Autodesk Fusion 360 part; units mm, degrees
sketch "Eskiz1" plane through (0, 0, 0) normal (0, 1, 0) x (1, 0, 0)
  circle A0 centre (0, 0) radius 20
  circle A1 centre (0, 0) radius 50
  line L0 (-5, 44.3809) -> (5, 44.3809)
  line L1 (5, 44.3809) -> (5, 24.3809)
  line L2 (5, 24.3809) -> (-5, 24.3809)
  line L3 (-5, 24.3809) -> (-5, 44.3809)
  circle A2 centre (-5, 24.3809) radius 1.5
  circle A3 centre (5, 24.3809) radius 1.5
  circle A4 centre (-5, 44.3809) radius 1.5
  circle A5 centre (5, 44.3809) radius 1.5
  circle A6 centre (-34.9176, 27.8465) radius 1.5
  line L4 (-34.9176, 27.8465) -> (-27.8465, 34.9176)
  line L5 (-20.7754, 13.7044) -> (-34.9176, 27.8465)
  line L6 (-13.7044, 20.7754) -> (-20.7754, 13.7044)
  line L7 (-27.8465, 34.9176) -> (-13.7044, 20.7754)
  circle A7 centre (-27.8465, 34.9176) radius 1.5
  circle A8 centre (-20.7754, 13.7044) radius 1.5
  circle A9 centre (-13.7044, 20.7754) radius 1.5
  circle A10 centre (-44.3809, -5) radius 1.5
  line L8 (-44.3809, -5) -> (-44.3809, 5)
  line L9 (-24.3809, -5) -> (-44.3809, -5)
  line L10 (-24.3809, 5) -> (-24.3809, -5)
  line L11 (-44.3809, 5) -> (-24.3809, 5)
  circle A11 centre (-44.3809, 5) radius 1.5
  circle A12 centre (-24.3809, -5) radius 1.5
  circle A13 centre (-24.3809, 5) radius 1.5
  circle A14 centre (-27.8465, -34.9176) radius 1.5
  line L12 (-27.8465, -34.9176) -> (-34.9176, -27.8465)
  line L13 (-13.7044, -20.7754) -> (-27.8465, -34.9176)
  line L14 (-20.7754, -13.7044) -> (-13.7044, -20.7754)
  line L15 (-34.9176, -27.8465) -> (-20.7754, -13.7044)
  circle A15 centre (-34.9176, -27.8465) radius 1.5
  circle A16 centre (-13.7044, -20.7754) radius 1.5
  circle A17 centre (-20.7754, -13.7044) radius 1.5
  circle A18 centre (5, -44.3809) radius 1.5
  line L16 (5, -44.3809) -> (-5, -44.3809)
  line L17 (5, -24.3809) -> (5, -44.3809)
  line L18 (-5, -24.3809) -> (5, -24.3809)
  line L19 (-5, -44.3809) -> (-5, -24.3809)
  circle A19 centre (-5, -44.3809) radius 1.5
  circle A20 centre (5, -24.3809) radius 1.5
  circle A21 centre (-5, -24.3809) radius 1.5
  circle A22 centre (34.9176, -27.8465) radius 1.5
  line L20 (34.9176, -27.8465) -> (27.8465, -34.9176)
  line L21 (20.7754, -13.7044) -> (34.9176, -27.8465)
  line L22 (13.7044, -20.7754) -> (20.7754, -13.7044)
  line L23 (27.8465, -34.9176) -> (13.7044, -20.7754)
  circle A23 centre (27.8465, -34.9176) radius 1.5
  circle A24 centre (20.7754, -13.7044) radius 1.5
  circle A25 centre (13.7044, -20.7754) radius 1.5
  circle A26 centre (44.3809, 5) radius 1.5
  line L24 (44.3809, 5) -> (44.3809, -5)
  line L25 (24.3809, 5) -> (44.3809, 5)
  line L26 (24.3809, -5) -> (24.3809, 5)
  line L27 (44.3809, -5) -> (24.3809, -5)
  circle A27 centre (44.3809, -5) radius 1.5
  circle A28 centre (24.3809, 5) radius 1.5
  circle A29 centre (24.3809, -5) radius 1.5
  circle A30 centre (27.8465, 34.9176) radius 1.5
  line L28 (27.8465, 34.9176) -> (34.9176, 27.8465)
  line L29 (13.7044, 20.7754) -> (27.8465, 34.9176)
  line L30 (20.7754, 13.7044) -> (13.7044, 20.7754)
  line L31 (34.9176, 27.8465) -> (20.7754, 13.7044)
  circle A31 centre (34.9176, 27.8465) radius 1.5
  circle A32 centre (13.7044, 20.7754) radius 1.5
  circle A33 centre (20.7754, 13.7044) radius 1.5
  circle A34 centre (0, 0) radius 3.9
  point P0 (-5, 0)
  point P1 (5, 0)
  dimension "d1" = 40
  dimension "d2" = 100
  dimension "d3" = 5
  dimension "d4" = 5
  dimension "d5" = 10
  dimension "d6" = 20
  dimension "d9" = 44.3809
  dimension "d10" = 3
  dimension "d11" = 3
  dimension "d12" = 3
  dimension "d13" = 3
  dimension "d15" = 360
  dimension "d16" = 7.8
extrude "Ekstrüde Et1" add sketch "Eskiz1" along normal blind 10 contours A0 | A1
extrude "Ekstrüde Et2" add sketch "Eskiz1" along normal blind 6.5 contours A0
sketch "Eskiz2" plane through (0, 10, 0) normal (0, 1, 0) x (-1, 0, 0)
  arc A0 (-14.765, -21.8361) -> (-14.765, -19.7148) centre (-13.7044, -20.7754) ccw
  line L0 (-14.765, -21.8361) -> (-26.7858, -33.8569)
  arc A1 (-28.9072, -33.8569) -> (-26.7858, -33.8569) centre (-27.8465, -34.9176) ccw
  line L1 (-28.9072, -33.8569) -> (-33.8569, -28.9072)
  arc A2 (-33.8569, -26.7858) -> (-33.8569, -28.9072) centre (-34.9176, -27.8465) ccw
  line L2 (-33.8569, -26.7858) -> (-21.8361, -14.765)
  arc A3 (-19.7148, -14.765) -> (-21.8361, -14.765) centre (-20.7754, -13.7044) ccw
  line L3 (-19.7148, -14.765) -> (-14.765, -19.7148)
  circle A4 centre (0, 0) radius 3.9
  arc A5 (-3.5, -24.3809) -> (-5, -25.8809) centre (-5, -24.3809) ccw
  line L4 (-3.5, -24.3809) -> (3.5, -24.3809)
  arc A6 (5, -25.8809) -> (3.5, -24.3809) centre (5, -24.3809) ccw
  line L5 (5, -25.8809) -> (5, -42.8809)
  arc A7 (3.5, -44.3809) -> (5, -42.8809) centre (5, -44.3809) ccw
  line L6 (3.5, -44.3809) -> (-3.5, -44.3809)
  arc A8 (-5, -42.8809) -> (-3.5, -44.3809) centre (-5, -44.3809) ccw
  line L7 (-5, -42.8809) -> (-5, -25.8809)
  arc A9 (21.8361, -14.765) -> (19.7148, -14.765) centre (20.7754, -13.7044) ccw
  line L8 (21.8361, -14.765) -> (33.8569, -26.7858)
  arc A10 (33.8569, -28.9072) -> (33.8569, -26.7858) centre (34.9176, -27.8465) ccw
  line L9 (33.8569, -28.9072) -> (28.9072, -33.8569)
  arc A11 (26.7858, -33.8569) -> (28.9072, -33.8569) centre (27.8465, -34.9176) ccw
  line L10 (26.7858, -33.8569) -> (14.765, -21.8361)
  arc A12 (14.765, -19.7148) -> (14.765, -21.8361) centre (13.7044, -20.7754) ccw
  line L11 (14.765, -19.7148) -> (19.7148, -14.765)
  arc A13 (25.8809, 5) -> (24.3809, 3.5) centre (24.3809, 5) ccw
  line L12 (25.8809, 5) -> (42.8809, 5)
  arc A14 (44.3809, 3.5) -> (42.8809, 5) centre (44.3809, 5) ccw
  line L13 (44.3809, 3.5) -> (44.3809, -3.5)
  arc A15 (42.8809, -5) -> (44.3809, -3.5) centre (44.3809, -5) ccw
  line L14 (42.8809, -5) -> (25.8809, -5)
  arc A16 (24.3809, -3.5) -> (25.8809, -5) centre (24.3809, -5) ccw
  line L15 (24.3809, -3.5) -> (24.3809, 3.5)
  arc A17 (14.765, 21.8361) -> (14.765, 19.7148) centre (13.7044, 20.7754) ccw
  line L16 (14.765, 21.8361) -> (26.7858, 33.8569)
  arc A18 (28.9072, 33.8569) -> (26.7858, 33.8569) centre (27.8465, 34.9176) ccw
  line L17 (28.9072, 33.8569) -> (33.8569, 28.9072)
  arc A19 (33.8569, 26.7858) -> (33.8569, 28.9072) centre (34.9176, 27.8465) ccw
  line L18 (33.8569, 26.7858) -> (21.8361, 14.765)
  arc A20 (19.7148, 14.765) -> (21.8361, 14.765) centre (20.7754, 13.7044) ccw
  line L19 (19.7148, 14.765) -> (14.765, 19.7148)
  arc A21 (-5, 25.8809) -> (-3.5, 24.3809) centre (-5, 24.3809) ccw
  line L20 (-5, 25.8809) -> (-5, 42.8809)
  arc A22 (-3.5, 44.3809) -> (-5, 42.8809) centre (-5, 44.3809) ccw
  line L21 (-3.5, 44.3809) -> (3.5, 44.3809)
  arc A23 (5, 42.8809) -> (3.5, 44.3809) centre (5, 44.3809) ccw
  line L22 (5, 42.8809) -> (5, 25.8809)
  arc A24 (3.5, 24.3809) -> (5, 25.8809) centre (5, 24.3809) ccw
  line L23 (3.5, 24.3809) -> (-3.5, 24.3809)
  arc A25 (-33.8569, 28.9072) -> (-33.8569, 26.7858) centre (-34.9176, 27.8465) ccw
  line L24 (-33.8569, 28.9072) -> (-28.9072, 33.8569)
  arc A26 (-26.7858, 33.8569) -> (-28.9072, 33.8569) centre (-27.8465, 34.9176) ccw
  line L25 (-26.7858, 33.8569) -> (-14.765, 21.8361)
  arc A27 (-14.765, 19.7148) -> (-14.765, 21.8361) centre (-13.7044, 20.7754) ccw
  line L26 (-14.765, 19.7148) -> (-19.7148, 14.765)
  arc A28 (-21.8361, 14.765) -> (-19.7148, 14.765) centre (-20.7754, 13.7044) ccw
  line L27 (-21.8361, 14.765) -> (-33.8569, 26.7858)
  arc A29 (-44.3809, -3.5) -> (-42.8809, -5) centre (-44.3809, -5) ccw
  line L28 (-44.3809, -3.5) -> (-44.3809, 3.5)
  arc A30 (-42.8809, 5) -> (-44.3809, 3.5) centre (-44.3809, 5) ccw
  line L29 (-42.8809, 5) -> (-25.8809, 5)
  arc A31 (-24.3809, 3.5) -> (-25.8809, 5) centre (-24.3809, 5) ccw
  line L30 (-24.3809, 3.5) -> (-24.3809, -3.5)
  arc A32 (-25.8809, -5) -> (-24.3809, -3.5) centre (-24.3809, -5) ccw
  line L31 (-25.8809, -5) -> (-42.8809, -5)
  circle A33 centre (0, 0) radius 50
Geometry: final body of the model. Coordinates: model frame, mm. Round coordinates to 2 decimals unless told otherwise and drop trailing zeros. Loops run counter-clockwise (first coordinate to the right, second up) from the corner with the lowest first, then second, coordinate; pieces in that order, holes last. Notation, with made-up numbers: M -4,35.25 L 25,35.25 A26 ccw 25,57.25 Z; hole C -4.5,72 d6. An arc over 180 degrees is marked long. Put each result on its own line as item: value. Start each with the question number.
(1) Section query B-B (x = 0). Return loops of the section in (y, z), then the cut area to 3 significant figures.
(2) Contact query for flat-ended pins moving along their axis: pin 1 Ø3 at (y, z) = (4.5, 35) entering from +X; pin 2 Ø1 at (x, y) = (26, 3) entering from +Z; pin 3 Ø5 at (y, z) = (4, -31.5) entering from -X; pin 4 Ø2.5 at (x, z) = (-5, 24.38) entering from -Y. Output: stop coordinate, or through.
(3) Section query C-C (y = 5.5). State how many separate pieces and enclosed holes the cut face has, then the cut area to 3 significant figures.
(4) Draft query along X for faces 1 (the face through (0, 5, 24.381)), 2 (the face through (47.69, 4.93, 15.02)). Return one class per face: +X half, -X half, draft (parallel to the pull), parting line (faces both ways), or undercut.
(5) Section query A-A (z = 0). Return loops of the section in (x, y), then the cut area to 3 significant figures.
(6) Material intervals for line 1 along X through (y, z) = (6.5, 26.5); line 2 along X through (y, z) = (1.5, 14.5); line 3 along Z through (x, y) = (-29, 3.25), sorted ascending. Write a range as [from, to].
Findings below:
1. outline: M 0,-50 L 10,-50 L 10,-44.38 L 0,-44.38 Z; M 0,-24.38 L 10,-24.38 L 10,-3.9 L 0,-3.9 Z; M 0,3.9 L 10,3.9 L 10,24.38 L 0,24.38 Z; M 0,44.38 L 10,44.38 L 10,50 L 0,50 Z
1. area: 522 mm2
2. pin 1: stops at x = 37.12
2. pin 2: stops at z = 43.01
2. pin 3: stops at x = -40.73
2. pin 4: passes through
3. separate pieces: 1
3. enclosed holes: 9
3. area: 6,040 mm2
4. face 1: undercut
4. face 2: parting line
5. outline: M -50,0 L -44.38,0 L -44.38,10 L -50,10 Z; M -24.38,0 L -3.9,0 L -3.9,10 L -24.38,10 Z; M 3.9,0 L 24.38,0 L 24.38,10 L 3.9,10 Z; M 44.38,0 L 50,0 L 50,10 L 44.38,10 Z
5. area: 522 mm2
6. line 1: x = [-42.4, -35.58], [-34.26, -33.57], [-19.43, -5], [5, 19.43], [33.57, 34.26], [35.58, 42.4]
6. line 2: x = [-47.85, -22.05], [-19.5, 19.5], [22.05, 47.85]
6. line 3: z = [-40.73, -35.88], [-33.96, -33.76], [-21.93, -5], [5, 21.93], [33.76, 33.96], [35.88, 40.73]
